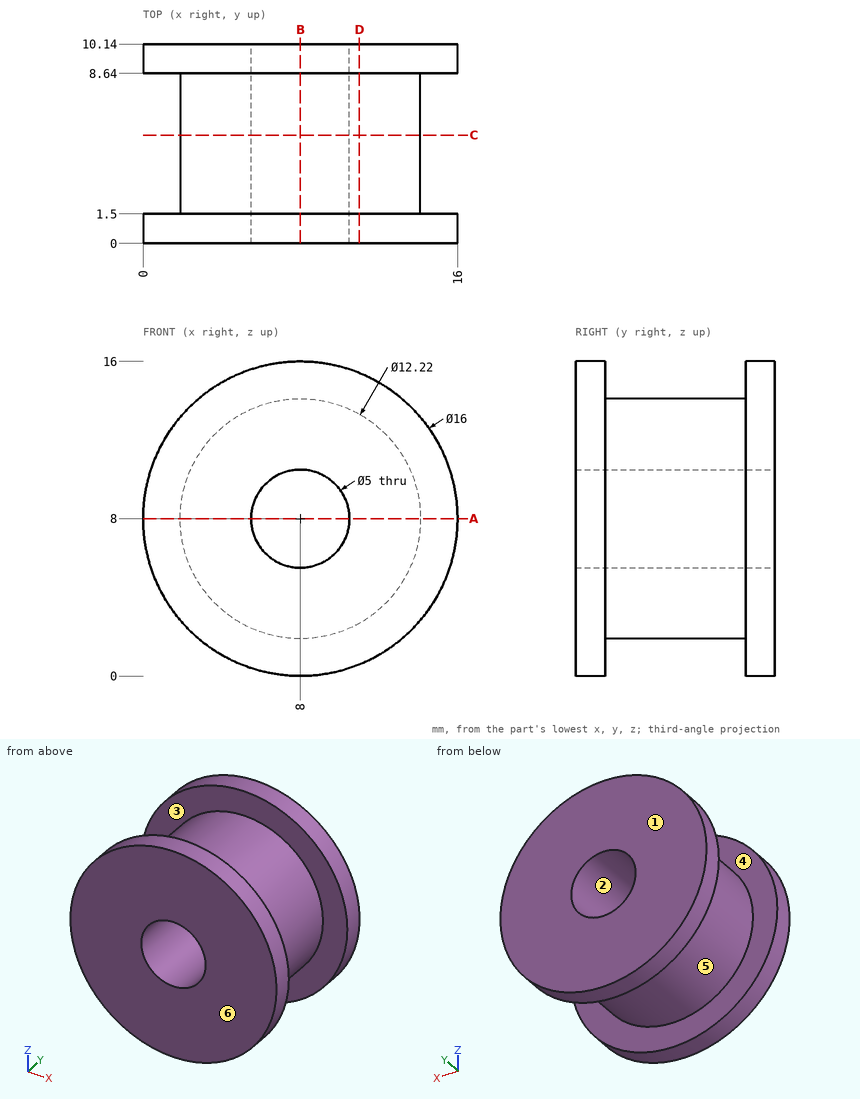
Design review of the part shown in the three views and the two pictorial views. Dimensions are in mm from the part's minimum x, y and z. A direction names the side the tool comes from. Give positions to 0.01 mm unless a question says otherwise; leave off trailing zeros. Loops run counter-clockwise (first coordinate to the right, second up) from the corner with the lowest first, then second, coordinate; pieces in that order, holes last. Notation, with made-up numbers: M 81.5,32.25 L 89.5,32.25 A10 cw 89.5,36.25 Z; hole C -26,89.25 d9. An arc over 180 degrees is marked long. Write item = value, one per line.
Q1. We need section B-B (x = 8). Give the boundary of the cut face in (y, z), plus the area to 3 significant figures.
Output values:
outline = M 0,0 L 1.5,0 L 1.5,1.89 L 8.64,1.89 L 8.64,0 L 10.14,0 L 10.14,5.5 L 0,5.5 Z; M 0,10.5 L 10.14,10.5 L 10.14,16 L 8.64,16 L 8.64,14.11 L 1.5,14.11 L 1.5,16 L 0,16 Z
area = 84.6 mm^2
Q2. Insertion check: pin 1 (8 mm diameter, centred on x = 8, z = 8, fed in from +Y); pin 2 (6 mm diameter, centred on y = 1, z = 12.5, fed in from -X); pin 3 (1.5 mm diameter, centred on x = 10, y = 5.5, fed in from -Z); pin 4 (3 mm diameter, centred on y = 6.5, z = 8, fed in from -X). Each pin has a flat end and moves straight along its axis. Give the tip position at first contact, or say it passes through.
Output values:
pin_1 = 10.14
pin_2 = 0.14
pin_3 = 2.02
pin_4 = 1.89
Q3. We need section C-C (y = 5.5). Give the boundary of the cut face in (x, z).
Output values:
outline = C 8,8 d12.22; hole C 8,8 d5
Q4. To check wall thickness, follow line 1 (Y direction, x = 10.25, z = 1); line 2 (Z direction, x = 8, y = 8). State the ranges of each line that lie inside material, in increasing order. Write a range as [from, to].
Output values:
line_1 = [0, 1.5], [8.64, 10.14]
line_2 = [1.89, 5.5], [10.5, 14.11]
Q5. For the marked faces 5 and 6, list the 3-axis set-ups (+Z, -Z, +X, -X, +Y, -Y) from which the entire face can be reached by the end or side of a thin tool; tool diameter is ignored.
Output values:
face_5 = none
face_6 = +Z, -Z, +X, -X, -Y
Q6. We need section D-D (x = 11). Give the boundary of the cut face in (y, z).
Output values:
outline = M 0,0.58 L 1.5,0.58 L 1.5,2.68 L 8.64,2.68 L 8.64,0.58 L 10.14,0.58 L 10.14,15.42 L 8.64,15.42 L 8.64,13.32 L 1.5,13.32 L 1.5,15.42 L 0,15.42 Z
Q7. We need section A-A (z = 8). Give the boundary of the cut face in (x, y).
Output values:
outline = M 0,0 L 5.5,0 L 5.5,10.14 L 0,10.14 L 0,8.64 L 1.89,8.64 L 1.89,1.5 L 0,1.5 Z; M 10.5,0 L 16,0 L 16,1.5 L 14.11,1.5 L 14.11,8.64 L 16,8.64 L 16,10.14 L 10.5,10.14 Z
Q8. Draft analysis for pull direction Y (two halves, no side actions). For the marked faces 1, 2, 3 and 4, state which applies: +Y half, -Y half, draft (parallel to the pull), parting line (faces both ways), or undercut.
Output values:
face_1 = +Y half
face_2 = draft
face_3 = undercut
face_4 = undercut
